from build123d import *

# Parameters (mm, degrees)
F0_R     = 40.915228
F0_R_2   = 28.015967
F1_DEPTH = 74.676
F2_DEPTH = 75.692
F3_R     = 55.991945
F3_R_2   = 28.179718
F4_DEPTH = 88.392
F6_R     = 33.015508
F7_DEPTH = 170.18


with BuildPart() as f1:
    # F0 (on Top) → F1 (new body)
    with BuildSketch(Plane.XY):
        Circle(F0_R)
        Circle(F0_R_2, mode=Mode.SUBTRACT)
    extrude(amount=F1_DEPTH)

    # F0 (on Top) → F2 (join)
    with BuildSketch(Plane.XY):
        Circle(F0_R)
        Circle(F0_R_2, mode=Mode.SUBTRACT)
    extrude(amount=-F2_DEPTH)

    # F3 (on Right) → F4 (join)
    with BuildSketch(Plane.YZ):
        Circle(F3_R)
        Circle(F3_R_2, mode=Mode.SUBTRACT)
    extrude(amount=F4_DEPTH)

    # F6 (on face) → F7 (cut)
    with BuildSketch(Plane.XY.offset(74.676)):
        with Locations((0, -17.064605)):
            Circle(F6_R)
    extrude(amount=-F7_DEPTH, mode=Mode.SUBTRACT)


solid = f1.part
Geometry: final body of the model. Coordinates: model frame, mm. A direction names the side the tool comes from. Coordinates: 2 decimals unless noted, no trailing zeros. Write each loop counter-clockwise with the first axis right and the second up, starting at its lowest first coordinate (ties: lowest second). Pieces come first, ordered by that corner, then holes. Notation, with made-up numbers: (80.25, 29) - (139.25, 29) arc R23 cw to (139.25, 52) - close; hole circle Ø7 at (53.5, 89.5). An arc over 180 degrees is marked (long way). Return JSON: item names as keys, results as strings.
Item 1: Section query A-A (z = 0). Output: boundary loops of the cut face in (x, y), and give its area (3 significant figures).
Completed:
{"outline": "(-31.88, -25.64) arc R33.02 cw to (-28.01, 0.41) arc R28.02 cw to (28.01, 0.41) arc R33.02 cw to (31.88, -25.64) arc R40.92 ccw to (29.66, 28.18) - (88.39, 28.18) - (88.39, 55.99) - (0, 55.99) - (0, 40.92) arc R40.92 ccw to start; (0, -55.99) - (88.39, -55.99) - (88.39, -28.18) - (31.09, -28.18) arc R33.02 cw to (0, -50.08) - close", "area": "5,870 mm2"}
Item 2: Line query: L1, parallel to Z at x = 65, y = 0; L2, parallel to X at y = 46, z = 12. Output: solid intervals per line, ascending.
Completed:
{"L1": "z = -55.99 to -28.18, 28.18 to 55.99", "L2": "x = 0 to 88.39"}
Item 3: Section query D-D (y = -7). Output: boundary loops of the cut face in (x, z), and give its area (3 significant figures).
Completed:
{"outline": "(-40.31, -75.69) - (-31.44, -75.69) - (-31.44, 74.68) - (-40.31, 74.68) - close; (31.44, -75.69) - (40.31, -75.69) - (40.31, -55.55) - (88.39, -55.55) - (88.39, -27.3) - (40.31, -27.3) - (40.31, 27.3) - (88.39, 27.3) - (88.39, 55.55) - (40.31, 55.55) - (40.31, 74.68) - (31.44, 74.68) - close", "area": "5,380 mm2"}
Item 4: Section query C-C (x = 48.5). Output: boundary loops of the cut face in (y, z), and give its area (3 significant figures).
Completed:
{"outline": "circle Ø111.98 at (0, 0); hole circle Ø56.36 at (0, 0)", "area": "7,350 mm2"}
Item 5: Pull-direction query (X, two-part tool) for faces 1 (the face through (0, 47, 1)), 2 (the face through (-8.92, 26.56, -1.56)), 3 (the face through (88.392, -26, -12)); classes: +X half, -X half, draft (parallel to the pull), parting line (faces both ways), or undercut.
Completed:
{"face 1": "-X half", "face 2": "undercut", "face 3": "+X half"}
Item 6: Reachability of faces 4 (the face through (10.698, 19.185, 20.641)), 5 (the face through (0, -52, 0)), 6 (the face through (53.4, 51.72, -21.45)), 7 (the face through (33.008, -17.791, 0.545)) from +Z, -Z, +X, -X, +Y, -Y: full face, straight path, thin tool, end or side. Return the list, or none.
Completed:
{"face 4": "none", "face 5": "+Z, -Z, -X, -Y", "face 6": "+X", "face 7": "+Z, -Z"}
Item 7: Pin query (flat end, axial travel): pin 1 Ø8 at (x, y) = (22.5, 41) entering from -Z; pin 2 Ø10 at (y, z) = (-23, -0.5) entering from -X; pin 3 Ø6 at (x, y) = (47.5, -13.5) entering from -Z. Return the tip coordinate at first contact, or that it passes through.
Completed:
{"pin 1": "stops at z = -42.02", "pin 2": "stops at x = -36.74", "pin 3": "stops at z = -55"}
Item 8: Section query B-B (y = 20). Output: boundary loops of the cut face in (x, z), and give its area (3 significant figures).
Completed:
{"outline": "(-35.69, -75.69) - (-19.62, -75.69) - (-19.62, 74.68) - (-35.69, 74.68) - close; (0, -52.3) - (19.62, -52.3) - (19.62, -75.69) - (35.69, -75.69) - (35.69, -52.3) - (88.39, -52.3) - (88.39, -19.85) - (35.69, -19.85) - (35.69, 19.85) - (88.39, 19.85) - (88.39, 52.3) - (35.69, 52.3) - (35.69, 74.68) - (19.62, 74.68) - (19.62, 52.3) - (0, 52.3) - (0, 19.85) - (19.62, 19.85) - (19.62, -19.85) - (0, -19.85) - close", "area": "9,530 mm2"}
